Source: three-view drawing plus pictorial views. Frame: mm from the lowest corner of the part. A direction names the side the tool comes from. Round coordinates to 2 decimals unless told otherwise and drop trailing zeros. Loops run counter-clockwise (first coordinate to the right, second up) from the corner with the lowest first, then second, coordinate; pieces in that order, holes last. Notation, with made-up numbers: (-27.75, 3.25) -> (1.25, 3.25) arc R28 ccw to (1.25, 26.25) -> close; hole circle Ø3 at (-13, 61.25). An arc over 180 degrees is marked (long way). Answer in a Markdown table with one row per item.
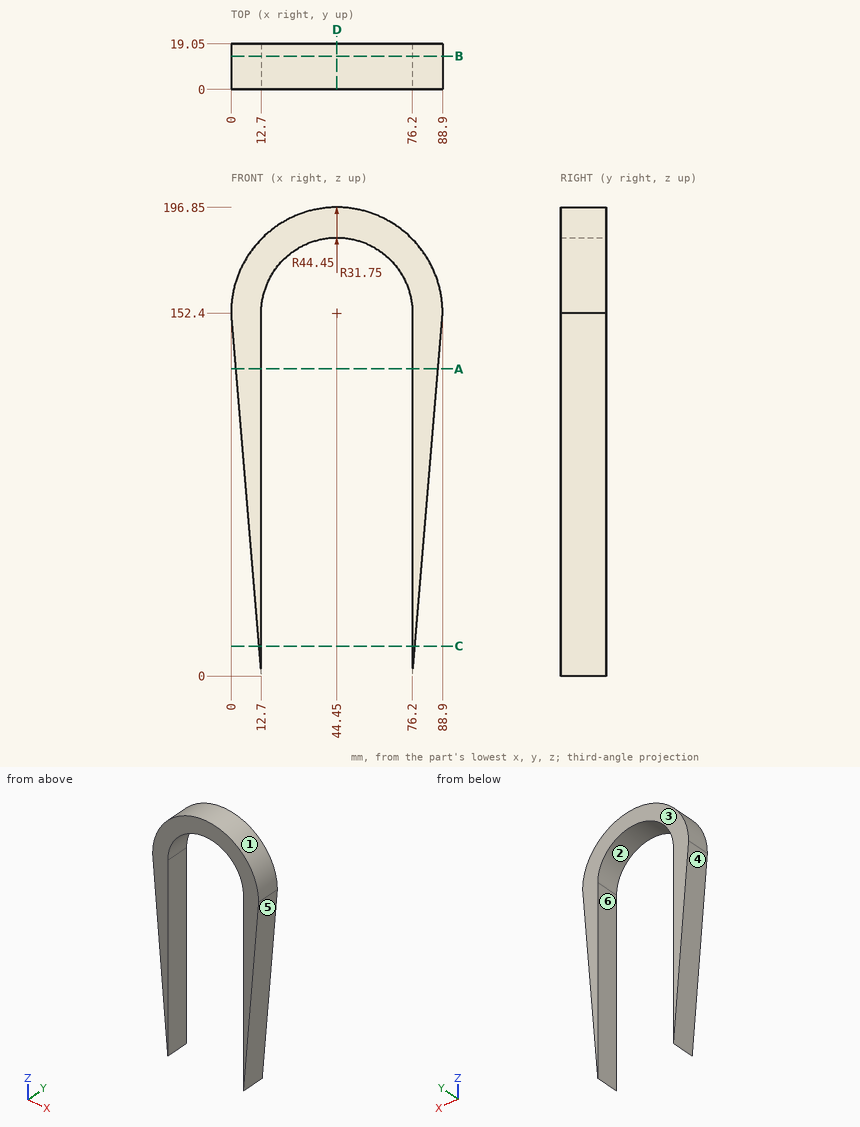
Item 1: Line query: probe 1 along X at (y, z) = (17, 149); probe 2 along X at (y, z) = (2.25, 166.5); probe 3 along Z at (x, y) = (57.5, 14.5). Output: solid intervals per line, ascending. Write a range as [from, to].
Answer:
| item | result |
|---|---|
| probe 1 | x = [0.28, 12.7], [76.2, 88.62] |
| probe 2 | x = [2.3, 16], [72.9, 86.6] |
| probe 3 | z = [181.34, 194.89] |
Item 2: Cut plane A-A (z = 129). Output: boundary loops of the cut face in (x, y).
Answer:
| item | result |
|---|---|
| outline | (1.95, 0) -> (12.7, 0) -> (12.7, 19.05) -> (1.95, 19.05) -> close; (76.2, 0) -> (86.95, 0) -> (86.95, 19.05) -> (76.2, 19.05) -> close |
Item 3: Cut plane D-D (x = 44.45). Output: boundary loops of the cut face in (y, z).
Answer:
| item | result |
|---|---|
| outline | (0, 184.15) -> (19.05, 184.15) -> (19.05, 196.85) -> (0, 196.85) -> close |
Item 4: Pin query (flat end, axial travel): pin 1 Ø3 at (y, z) = (9.5, 164.5) entering from +X; pin 2 Ø3 at (y, z) = (4.5, 171) entering from -X; pin 3 Ø6 at (y, z) = (11.5, 67.5) entering from -X (3 decimals). Return the tip coordinate at first contact, or that it passes through.
Answer:
| item | result |
|---|---|
| pin 1 | stops at x = 87.62 |
| pin 2 | stops at x = 3.42 |
| pin 3 | stops at x = 6.825 |
Item 5: Cut plane B-B (y = 14). Output: boundary loops of the cut face in (x, z).
Answer:
| item | result |
|---|---|
| outline | (0, 152.4) -> (12.7, 0) -> (12.7, 152.4) arc R31.75 cw to (76.2, 152.4) -> (76.2, 0) -> (88.9, 152.4) arc R44.45 ccw to start |
Item 6: Draft query along X for the marked faces 1, 2, 3 and 4. Return one class per face: pulls with the +X half, pulls with the -X half, needs draft (parallel to the pull), parting line crosses it, or undercut.
Answer:
| item | result |
|---|---|
| face 1 | parting line crosses it |
| face 2 | undercut |
| face 3 | needs draft |
| face 4 | pulls with the -X half |
Item 7: Cut plane C-C (z = 12.5). Output: boundary loops of the cut face in (x, y), then the cut area to 3 significant figures.
Answer:
| item | result |
|---|---|
| outline | (11.66, 0) -> (12.7, 0) -> (12.7, 19.05) -> (11.66, 19.05) -> close; (76.2, 0) -> (77.24, 0) -> (77.24, 19.05) -> (76.2, 19.05) -> close |
| area | 39.7 mm² |
Item 8: Reachability of the marked faces 5 and 6 from +Z, -Z, +X, -X, +Y, -Y: full face, straight path, thin tool, end or side. Return the list, or none.
Answer:
| item | result |
|---|---|
| face 5 | -Z, +X, +Y, -Y |
| face 6 | -Z, +Y, -Y |
